Input: part model. Units: mm. Frame: model coordinates. A direction names the side the tool comes from. Round coordinates to 2 decimals unless told otherwise and drop trailing zeros. Loops run counter-clockwise (first coordinate to the right, second up) from the corner with the lowest first, then second, coordinate; pieces in that order, holes last. Notation, with made-up numbers: (87.25, 63.5) -> (141.25, 63.5) arc R26 ccw to (141.25, 87.5) -> close; hole circle Ø8 at (83.25, 60.25). An arc over 180 degrees is marked (long way). Answer in a Markdown table with one row per item. Add a question column.
Q1. Section B-B, the plane y = -2. Output: boundary loops of the cut face in (x, z), and give its area (3 significant figures).
Q2. Ray query, L1, parallel to Z at x = 0, y = -9.5; L2, parallel to Z at x = 1, y = -6.25; L3, parallel to Y at x = -4, z = -0.5. Return the intervals inside material, ascending. Write a range as from..to.
Q3. Mould query, pull axis Z, two halves, no side actions, for faces 1 (the face through (3.2, -14.93, 2.27)), 2 (the face through (-0.54, -7.4, -2.44)), 3 (the face through (3.609, -12.468, -1.726)), 4 (the face through (1, -15, 3)). Classes: pulls with the +Z half, pulls with the -Z half, needs draft (parallel to the pull), parting line crosses it, or undercut.
Q4. Pin query (flat end, axial travel): pin 1 (1 mm diameter, centred on y = -2.5, z = -2.5, fed in from +X); pin 2 (2 mm diameter, centred on y = -12.5, z = 3, fed in from +X); pin 3 (2 mm diameter, centred on y = -2.5, z = 3, fed in from -X). Return the tip coordinate at first contact, or that it passes through.
Q5. Section A-A, the plane y = -11.5. Output: boundary loops of the cut face in (x, z), and give its area (3 significant figures).
Q6. Reachability of faces 5 (the face through (3.57, -14.925, -1.641)), 6 (the face through (3.233, -4.933, -1.341)) from +Z, -Z, +X, -X, +Y, -Y: full face, straight path, thin tool, end or side. Return the list, or none.
```python
from build123d import *

# Parameters (mm, degrees)
F0_R     = 3.5
F0_R_2   = 2.5
F1_DEPTH = 10
F2_START = 10
F2_DEPTH = 5
F3_R     = 0.24999


# Not quite as in the source:
# - a fillet or chamfer is up to 0.001 mm smaller than in the source, because OpenCascade refuses the exact size


with BuildPart() as f1:
    # F0 (on Front) → F1 (new body)
    with BuildSketch(Plane.XZ):
        Circle(F0_R)
        Circle(F0_R_2, mode=Mode.SUBTRACT)
    extrude(amount=F1_DEPTH)

    # F0 (on Front) → F2 (join)
    with BuildSketch(Plane.XZ.offset(F2_START)):
        Polygon((2.6409240726, -3.78930777), (4.6020988279, 0.3924534514), (1.9611747553, 4.1817612214), (-2.6409240726, 3.78930777), (-4.6020988279, -0.3924534514), (-1.9611747553, -4.1817612214), align=None)
        Circle(F0_R, mode=Mode.SUBTRACT)
        Circle(F0_R)
        Circle(F0_R_2, mode=Mode.SUBTRACT)
    extrude(amount=F2_DEPTH)

    # F3 (radius 0.25 in the source; OpenCascade refuses exactly that, so slightly less here)
    f3_edges = [f1.edges().sort_by_distance(p)[0] for p in [
        (-2.5, -15, 0),
        (-0.339875, -15, 3.985534),
        (-0.339875, -10, 3.985534),
        (1.961175, -12.5, 4.181761),
        (-3.5, 0, 0),
        (-2.640924, -12.5, 3.789308),
        (-3.621511, -15, 1.698427),
        (-3.281637, -15, -2.287107),
        (-3.621511, -10, 1.698427),
        (-3.281637, -10, -2.287107),
        (-1.961175, -12.5, -4.181761),
        (0.339875, -10, -3.985534),
        (2.640924, -12.5, -3.789308),
        (0.339875, -15, -3.985534),
        (3.621511, -15, -1.698427),
        (3.281637, -15, 2.287107),
        (4.602099, -12.5, 0.392453),
        (3.621511, -10, -1.698427),
        (3.281637, -10, 2.287107),
        (-3.5, -10, 0),
        (-2.5, 0, 0),
    ]]
    fillet(f3_edges, radius=F3_R)


solid = f1.part
```
Answer block:
| question | item | result |
|---|---|---|
| 1 | outline | circle Ø7 at (0, 0); hole circle Ø5 at (0, 0) |
| 1 | area | 18.8 mm^2 |
| 2 | L1 | -3.5..-2.5, 2.5..3.5 |
| 2 | L2 | -3.35..-2.29, 2.29..3.35 |
| 2 | L3 | -15..-10 |
| 3 | face 1 | pulls with the +Z half |
| 3 | face 2 | undercut |
| 3 | face 3 | pulls with the -Z half |
| 3 | face 4 | needs draft |
| 4 | pin 1 | x = 2.87 |
| 4 | pin 2 | x = 3.48 |
| 4 | pin 3 | x = -2.87 |
| 5 | outline | (-4.6, -0.39) -> (-2.04, -4.06) arc R0.25 ccw to (-1.82, -4.17) -> (2.5, -3.8) arc R0.25 ccw to (2.7, -3.66) -> (4.54, 0.26) arc R0.25 ccw to (4.52, 0.51) -> (2.04, 4.06) arc R0.25 ccw to (1.82, 4.17) -> (-2.5, 3.8) arc R0.25 ccw to (-2.7, 3.66) -> close; hole circle Ø5 at (0, 0) |
| 5 | area | 35.8 mm^2 |
| 6 | face 5 | -Z, +X, -Y |
| 6 | face 6 | +Y |
